The listing builds one solid part. Answer for the finished solid, in the listing's coordinates (mm). Coordinates: 2 decimals unless noted, no trailing zeros. One line per question, with ' | ' between items.
from build123d import *


with BuildPart() as part:
    # Çizim2 → Döndür4 (revolve)
    with BuildSketch(Plane.XY, mode=Mode.PRIVATE) as d_nd_r4_sk:
        with BuildLine():
            Line((0.007868423, 2.447551496), (0, 0))
            Line((0, 0), (0.029070392, 0))
            ThreePointArc((0.029070392, 0), (6.663636067, 0.442575925), (13.180632211, 1.762460918))
            Line((13.180632211, 1.762460918), (13.025393844, 4.311738481))
            Line((13.025393844, 4.311738481), (12.905238293, 4.277863766))
            ThreePointArc((12.905238293, 4.277863766), (8.500440894, 3.259791078), (4.018750105, 2.665518584))
            Line((4.018750105, 2.665518584), (4.018750105, 2.447549997))
            Line((4.018750105, 2.447549997), (0.007868423, 2.447551496))
        make_face()
    revolve(d_nd_r4_sk.sketch.rotate(Axis((0.007868423, 2.447551496, 0), (-0.0032147973142897033, -0.9999948325257627, 0)), 180), axis=Axis((0.007868423, 2.447551496, 0), (-0.0032147973142897033, -0.9999948325257627, 0)))


solid = part.part
Item 1: Each of these flat-tipped pins is pushed along its axis until it touches: pin 1 Ø12 at (x, z) = (-5.5, 2.5) entering from -Y; pin 2 Ø1.5 at (x, y) = (-4, 2) entering from +Z; pin 3 Ø2 at (x, y) = (5, 2) entering from +Z; pin 4 Ø2 at (x, z) = (3.5, -9) entering from +Y. Where does it stop, or does it pass through?
Computed values:
pin 1: stops at y = 0 | pin 2: stops at z = 12.76 | pin 3: stops at z = 12.55 | pin 4: stops at y = 3.73
Item 2: Find the intervals of material crossed by L1, parallel to Z at x = -3.5, y = 2.6; L2, parallel to Y at x = -1.75, z = 12; L3, parallel to Y at x = 4.5, z = 2.25, in increasing order.
Computed values:
L1: z = -12.65 to -1.94, 1.94 to 12.65 | L2: y = 1.53 to 4.11 | L3: y = 0.25 to 2.76
Item 3: Determine the mould class of faces 1 (the face through (1.71, 3.941, -12.927)), 2 (the face through (0.05, 2.45, 0.19)) for opening direction Z: pulls with the +Z half, pulls with the -Z half, needs draft (parallel to the pull), parting line crosses it, or undercut.
Computed values:
face 1: parting line crosses it | face 2: undercut
